from build123d import *

# Parameters (mm, degrees)
BOSS_EXTRUDE2_DEPTH = 3
CUT_EXTRUDE1_DEPTH  = 10
FILLET1_R           = 5
FILLET2_R           = 5


with BuildPart() as part:
    # Sketch1 → Boss-Extrude2 (new body)
    with BuildSketch(Plane(origin=(0, 0, 0), x_dir=(1, 0, 0), z_dir=(0, 1, 0))):
        Polygon((37, 220), (67, 220), (67, 180), (37, 180), (37, -220), (-37, -220), (-37, 220), align=None)
    extrude(amount=BOSS_EXTRUDE2_DEPTH)

    # Sketch3 → 3/8-16 Tapped Hole1 (revolve, cut)
    with BuildSketch(Plane(origin=(54, 3, -200), x_dir=(0, 0, 1), z_dir=(1, 0, 0))):
        Polygon((0, 0), (0, 3), (3.96875, 3), (3.96875, 1.198863598), (5.3975, 0), align=None)
    revolve(axis=Axis((54, 9.35, -200), (0, -1, 0)), mode=Mode.SUBTRACT)

    # Sketch5 → Cut-Extrude1 (cut)
    with BuildSketch(Plane.XZ):
        Polygon((37, 220), (37, 211.960805492), (22.794358884, 220), align=None)
    extrude(amount=-CUT_EXTRUDE1_DEPTH, mode=Mode.SUBTRACT)

    # Fillet1
    fillet1_edges = [part.edges().sort_by_distance(p)[0] for p in [
        (37, 1.5, 211.960805492),
    ]]
    fillet(fillet1_edges, radius=FILLET1_R)

    # Fillet2
    fillet2_edges = [part.edges().sort_by_distance(p)[0] for p in [
        (22.794358884, 1.5, 220),
    ]]
    fillet(fillet2_edges, radius=FILLET2_R)


solid = part.part
For this review, take the finished solid that the model builds, in its own axes (mm). Coordinates: 2 decimals unless noted, no trailing zeros. Order: outer loops, then holes, each group sorted by start corner. A loop starts at its lowest first (then second) coordinate and runs counter-clockwise, first axis right, second up. Notation, with made-up numbers: (35, 10.25) - (56, 10.25) arc R25 ccw to (56, 31.25) - close; hole circle Ø1 at (-4.75, 47.25). An arc over 180 degrees is marked (long way). Use one line per item in the form item = value.
Q1. Consider section C-C (y = 1.1). Give the boundary of the cut face in (x, z).
Checked values:
outline = (-37, -220) - (67, -220) - (67, -180) - (37, -180) - (37, 209.05) arc R5 ccw to (34.46, 213.4) - (23.94, 219.35) arc R5 ccw to (21.48, 220) - (-37, 220) - close; hole circle Ø7.94 at (54, -200)
Q2. Draft analysis for pull direction X (two halves, no side actions). For faces 1 (the cylindrical face through (52.808, 0.913, -196.215)), 2 (the flat face through (4, 0, -3)), state which applies: +X half, -X half, draft (parallel to the pull), parting line (faces both ways), or undercut.
Checked values:
face_1 = undercut
face_2 = draft
Q3. Consider section A-A (z = -200). Give the boundary of the cut face in (x, y).
Checked values:
outline = (-37, 0) - (50.03, 0) - (50.03, 1.8) - (48.6, 3) - (-37, 3) - close; (57.97, 0) - (67, 0) - (67, 3) - (59.4, 3) - (57.97, 1.8) - close
Q4. Consider section B-B (x = 54). Give the boundary of the cut face in (y, z), then the cut area to 3 significant figures.
Checked values:
outline = (0, -220) - (3, -220) - (3, -205.4) - (1.8, -203.97) - (0, -203.97) - close; (0, -196.03) - (1.8, -196.03) - (3, -194.6) - (3, -180) - (0, -180) - close
area = 94.5 mm2
Q5. For probe 1 along X at (y, z) = (0.65, -200); probe 2 along Z at (x, y) = (54, 0.8); probe 3 along X at (y, z) = (0.85, 6.5), list the stretches that pass through material, from the lowest coordinate up. Write a range as from..to.
Checked values:
probe_1 = -37..50.03, 57.97..67
probe_2 = -220..-203.97, -196.03..-180
probe_3 = -37..37
Q6. Consider section D-D (z = -38). Give the boundary of the cut face in (x, y), then the cut area to 3 significant figures.
Checked values:
outline = (-37, 0) - (37, 0) - (37, 3) - (-37, 3) - close
area = 222 mm2
Q7. For P1, Ø1.5, axis at y = 2, z = 36.5, coming from the +X side, flat-tipped, find the tip position at first contact; note if it passes through.
Checked values:
P1 = 37
